Part model, mm, in its own coordinate system. A direction names the side the tool comes from. Coordinates: 2 decimals unless noted, no trailing zeros. Write each loop counter-clockwise with the first axis right and the second up, starting at its lowest first coordinate (ties: lowest second). Pieces come first, ordered by that corner, then holes. Notation, with made-up numbers: M -34.75,49 L 4.25,49 A21 ccw 4.25,64 Z; hole C 65.25,72 d2. An arc over 180 degrees is marked long. Use a Markdown table: item, result. Add a question column.
Q1. Slice it at C-C on z = 701.5. Write the cut outline in (x, y).
Q2. Pin check, flat tips, straight feed: pin 1 Ø10 at (y, z) = (47.5, 671) entering from +X; pin 2 Ø8 at (x, z) = (22.5, 562) entering from +Y. Stop position of each tip, or through.
Q3. Slice it at D-D on x = 22. Write the cut outline in (y, z).
Q4. Slice it at B-B on y = 50.8. Write the cut outline in (x, z).
Q5. Wall check: L1, parallel to Z at x = 2.75, y = 50.8; L2, parallel to Z at x = 3, y = 50; L3, parallel to Y at x = 4, z = 76.2. Give the ranges that are in metal, low to high. Write a range as from..to.
Q6. Tool access for faces 1 (the flat face through (5, 24, 0)), 2 (the flat face through (6.35, 44, 416)): list every direction of +Z, -Z, +X, -X, +Y, -Y with a clear straight run to the whole face (end or side of a thin tool).
Q7. Slice it at A-A on z = 76.2. Write the cut outline in (x, y).
Q8. Mould opens along Z. For faces 3 (the flat face through (5, 24, 844.55)), 4 (the cylindrical face through (3.131, 50.451, 430.205)), 5 (the flat face through (32, 6.35, 416)) say: released by +Z, released by -Z, zero draft, split by the parting line, or undercut.
Autodesk Inventor part; units mm, degrees
ref_plane "Start plane" through (0, 0, 0) normal (0, 0, 1) x (1, 0, 0)
ref_plane "End plane" through (0, 0, 844.55) normal (0, 0, 1) x (1, 0, 0)
ref_plane "YZ Plane" through (0, 0, 0) normal (1, 0, 0) x (0, 1, 0)
ref_plane "Start plane" through (0, 0, 0) normal (0, 0, 1) x (1, 0, 0)
ref_plane "End plane" through (0, 0, 844.55) normal (0, 0, 1) x (1, 0, 0)
sketch "Sketch" plane through (0, 0, 0) normal (0, 0, 1) x (1, 0, 0)
  line L0 (0, 76.2) -> (0, 0)
  line L1 (0, 0) -> (50.8, 0)
  line L2 (50.8, 0) -> (50.8, 4.35)
  line L3 (48.8, 6.35) -> (14.224, 6.35)
  line L4 (6.35, 14.224) -> (6.35, 74.2)
  line L5 (4.35, 76.2) -> (0, 76.2)
  line L6 (-7.0414, 0) -> (21.5385, 0) construction
  line L7 (0, -8.0414) -> (0, 34.5385) construction
  arc A0 (6.35, 14.224) -> (14.224, 6.35) centre (14.224, 14.224) ccw
  arc A1 (50.8, 4.35) -> (48.8, 6.35) centre (48.8, 4.35) ccw
  arc A2 (6.35, 74.2) -> (4.35, 76.2) centre (4.35, 74.2) ccw
  line L8 (0, 93.5453) -> (0, -24.9725) construction
  line L9 (-18.6925, 0) -> (62.8653, 0) construction
  point P0 (50.8, 6.35)
  point P1 (6.35, 6.35)
  point P2 (6.35, 76.2)
  dimension "d12" = 6.35
  dimension "d13" = 76.2
  dimension "d14" = 50.8
  dimension "d15" = 0
  dimension "d16" = 6.35
  dimension "d17" = 0
  dimension "d18" = 7.874
  dimension "d19" = 2
extrude "Body" add sketch "Sketch" along normal up to surface (844.55 mm away) from surface at 0
sketch "Sketch3" plane through (6.35, 14.224, 844.55) normal (1, 0, 0) x (0, 0, -1)
  line L0 (0, 59.976) -> (0, 0)
  line L1 (844.55, 59.976) -> (844.55, 0)
  line L2 (844.55, 59.976) -> (0, 59.976)
  line L3 (0, 36.576) -> (844.55, 36.576) construction
  line L4 (844.55, 61.976) -> (0, 61.976)
  point P0 (76.2, 36.576)
  point P1 (422.275, 36.576)
  point P2 (768.35, 36.576)
  dimension "d22" = 76.2
  dimension "d23" = 422.275
  dimension "d24" = 768.35
  dimension "d32" = 25.4
hole "Hole1" at (6.35, 50.8, 768.35) at (6.35, 50.8, 422.275) at (6.35, 50.8, 76.2) direction (-1, 0, 0) diameter 15.875 end through all
equation "\"d12\" = G_T"
equation "\"d13\" = G_H"
equation "\"d14\" = G_W"
equation "\"d16\" = G_T"
equation "\"d18\" = G_IR"
equation "\"d4\" = G_L"
equation "\"G_W\" = 50.8"
equation "\"G_H\" = 76.2"
equation "\"G_T\" = 6.35"
equation "\"G_ER\" = 4.064"
equation "\"G_IR\" = 7.874"
equation "\"G_L\" = B_L + G_OFFSET_START + G_OFFSET_END"
equation "\"ex\" = 0"
equation "\"ey\" = 0"
equation "\"G_OFFSET_START\" = 0"
equation "\"G_OFFSET_END\" = 0"
equation "\"d21\" = G_OFFSET_END + B_L"
equation "\"B_L\" = 844.55"
properties part number "ANSI L 3 x 2 x 1_4 00000011"
Recorded:
| question | item | result |
|---|---|---|
| 1 | outline | M 0,0 L 50.8,0 L 50.8,4.35 A2 ccw 48.8,6.35 L 14.22,6.35 A7.87 cw 6.35,14.22 L 6.35,74.2 A2 ccw 4.35,76.2 L 0,76.2 Z |
| 2 | pin 1 | x = 6.35 |
| 2 | pin 2 | y = 6.35 |
| 3 | outline | M 0,0 L 6.35,0 L 6.35,844.55 L 0,844.55 Z |
| 4 | outline | M 0,0 L 6.35,0 L 6.35,68.26 L 0,68.26 Z; M 0,84.14 L 6.35,84.14 L 6.35,414.34 L 0,414.34 Z; M 0,430.21 L 6.35,430.21 L 6.35,760.41 L 0,760.41 Z; M 0,776.29 L 6.35,776.29 L 6.35,844.55 L 0,844.55 Z |
| 5 | L1 | 0..68.26, 84.14..414.34, 430.21..760.41, 776.29..844.55 |
| 5 | L2 | 0..68.3, 84.1..414.38, 430.17..760.45, 776.25..844.55 |
| 5 | L3 | 0..42.86, 58.74..76.2 |
| 6 | face 1 | -Z, +X, -X, +Y, -Y |
| 6 | face 2 | +Z, -Z, +X, +Y |
| 7 | outline | M 0,0 L 50.8,0 L 50.8,4.35 A2 ccw 48.8,6.35 L 14.22,6.35 A7.87 cw 6.35,14.22 L 6.35,42.86 L 0,42.86 Z; M 0,58.74 L 6.35,58.74 L 6.35,74.2 A2 ccw 4.35,76.2 L 0,76.2 Z |
| 8 | face 3 | released by +Z |
| 8 | face 4 | undercut |
| 8 | face 5 | zero draft |
